from build123d import *

# Parameters (mm, degrees)
SKETCH1_W           = 1120
SKETCH1_H           = 40
BOSS_EXTRUDE1_DEPTH = 760
BOSS_EXTRUDE2_DEPTH = 1120
BOSS_EXTRUDE3_DEPTH = 1120
SKETCH4_W           = 137.769014226
SKETCH4_H           = 67.23794826
CUT_EXTRUDE1_DEPTH  = 1120


with BuildPart() as part:
    # Sketch1 → Boss-Extrude1 (new body)
    with BuildSketch(Plane(origin=(0, 0, 0), x_dir=(1, 0, 0), z_dir=(0, 1, 0))):
        Rectangle(SKETCH1_W, SKETCH1_H)
    extrude(amount=BOSS_EXTRUDE1_DEPTH)

    # Sketch2 → Boss-Extrude2 (add)
    with BuildSketch(Plane(origin=(560, 0, 0), x_dir=(0, 0, -1), z_dir=(1, 0, 0))):
        Polygon((-20, 760), (280, 1060), (320, 1060), (20, 760), align=None)
    extrude(amount=-BOSS_EXTRUDE2_DEPTH)

    # Sketch3 → Boss-Extrude3 (add)
    with BuildSketch(Plane(origin=(560, 0, 0), x_dir=(0, 0, -1), z_dir=(1, 0, 0))):
        Polygon((320, 1060), (1080, 1060), (1080, 1027), (285.570778589, 1027), align=None)
    extrude(amount=-BOSS_EXTRUDE3_DEPTH)

    # Sketch4 → Cut-Extrude1 (cut)
    with BuildSketch(Plane(origin=(0, 1060, 0), x_dir=(1, 0, 0), z_dir=(0, 1, 0))):
        with Locations((0, 1046.38102587)):
            Rectangle(SKETCH4_W, SKETCH4_H)
    extrude(amount=-CUT_EXTRUDE1_DEPTH, mode=Mode.SUBTRACT)


solid = part.part
Read the model definition and answer for the solid it produces. Units are mm, in the model's axes. A direction names the side the tool comes from. Give positions to 0.01 mm unless a question says otherwise; leave off trailing zeros. Write each loop counter-clockwise with the first axis right and the second up, starting at its lowest first coordinate (ties: lowest second). Pieces come first, ordered by that corner, then holes. Notation, with made-up numbers: (-9, -18) - (19, -18) arc R34 cw to (19, 15) - close; hole circle Ø10 at (7.5, 44). An arc over 180 degrees is marked (long way). Return JSON: item names as keys, results as strings.
Q1. A cutting plane is placed at A-A, the plane x = -41.5. Determine the outline of the cut face in (y, z), and give its area (3 significant figures).
Reply:
{"outline": "(0, -20) - (760, -20) - (1027, -287) - (1027, -1012.76) - (1060, -1012.76) - (1060, -280) - (760, 20) - (0, 20) - close", "area": "65,800 mm²"}
Q2. A cutting plane is placed at C-C, the plane z = -542.5. Determine the outline of the cut face in (x, y).
Reply:
{"outline": "(-560, 1027) - (560, 1027) - (560, 1060) - (-560, 1060) - close"}
Q3. For a pull along X with two mould halves and no side action, classify faces 4 (the face through (560, 925, -166)), 5 (the face through (-8, 375, 20)), 6 (the face through (-68.885, 1044, -1046)) as released by +X, released by -X, zero draft, split by the parting line, or undercut.
Reply:
{"face 4": "released by +X", "face 5": "zero draft", "face 6": "undercut"}
Q4. Consider line 1 along Y through (x, z) = (220.5, -938.5); line 2 along Z through (x, y) = (296, 43); line 3 along Y through (x, z) = (63, -165). Determine where each line is inside the solid, lowest interval first. Write a range as [from, to].
Reply:
{"line 1": "[1027, 1060]", "line 2": "[-20, 20]", "line 3": "[905, 945]"}
Q5. A cutting plane is placed at B-B, the plane y = 565. Determine the outline of the cut face in (x, z), and give its area (3 significant figures).
Reply:
{"outline": "(-560, -20) - (560, -20) - (560, 20) - (-560, 20) - close", "area": "44,800 mm²"}
Q6. A cutting plane is placed at D-D, the plane x = 371. Determine the outline of the cut face in (y, z).
Reply:
{"outline": "(0, -20) - (760, -20) - (1027, -287) - (1027, -1080) - (1060, -1080) - (1060, -280) - (760, 20) - (0, 20) - close"}
Q7. For faces 1 (the face through (68.885, 1044, -1046)), 2 (the face through (-311, 1044, -1080)), 3 (the face through (-8, 375, -20)), determine the directions among +Z, -Z, +X, -X, +Y, -Y from which every point of the face is accessible in a straight line to the end or side of a thin tool.
Reply:
{"face 1": "-Z, +Y, -Y", "face 2": "-Z, +X, -X, +Y, -Y", "face 3": "-Z, +X, -X, -Y"}
Q8. Given P1, Ø16.5, axis at x = 4, y = 1046, coming from the -Z side; P2, Ø2, axis at x = 145, z = -633, coming from the -Y side; P3, Ø8, axis at x = -367.5, z = -216.5, coming from the +Y side, each flat-ended and moving along its own axis, determine where each tip first touches the part or whether it passes through.
Reply:
{"P1": "z = -1012.76", "P2": "y = 1027", "P3": "y = 1000.5"}
